```python
from build123d import *

# Parameters (mm, degrees)
SKETCH1_R           = 1
BOSS_EXTRUDE1_DEPTH = 3
SKETCH2_R           = 1.25
CUT_EXTRUDE1_DEPTH  = 4
SKETCH3_R           = 1.25
CUT_EXTRUDE2_DEPTH  = 4


with BuildPart() as part:
    # Sketch1 → Boss-Extrude1 (new body)
    with BuildSketch(Plane(origin=(0, 2.5, 0), x_dir=(1, 0, 0), z_dir=(0, 1, 0))):
        with BuildLine():
            Line((-2.5, -48.662329453), (-2.5, -18.662329453))
            ThreePointArc((-2.5, -18.662329453), (-5, -16.162329453), (-7.5, -18.662329453))
            Line((-7.5, -18.662329453), (-7.5, -48.662329453))
            ThreePointArc((-7.5, -48.662329453), (-5, -51.162329453), (-2.5, -48.662329453))
        make_face()
        with Locations((-5, -48.662329453)):
            Circle(SKETCH1_R, mode=Mode.SUBTRACT)
        with Locations((-5, -18.662329453)):
            Circle(SKETCH1_R, mode=Mode.SUBTRACT)
    extrude(amount=-BOSS_EXTRUDE1_DEPTH)

    # Sketch2 → Cut-Extrude1 (cut, through all)
    with BuildSketch(Plane.XZ.offset(0.5)):
        with Locations((-5, 18.662329453)):
            Circle(SKETCH2_R)
    extrude(amount=-CUT_EXTRUDE1_DEPTH, mode=Mode.SUBTRACT)

    # Sketch3 → Cut-Extrude2 (cut, through all)
    with BuildSketch(Plane.XZ.offset(0.5)):
        with Locations((-5, 48.662329453)):
            Circle(SKETCH3_R)
    extrude(amount=-CUT_EXTRUDE2_DEPTH, mode=Mode.SUBTRACT)


solid = part.part
```
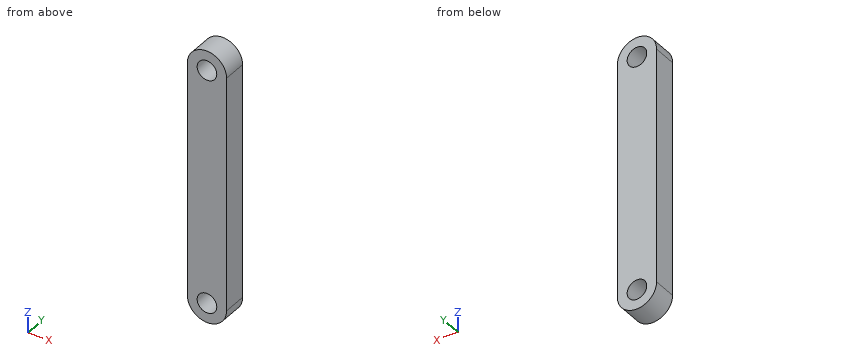
The model under review builds one solid part; all positions refer to its coordinate system, in mm. Round coordinates to 2 decimals unless told otherwise and drop trailing zeros. Loops run counter-clockwise (first coordinate to the right, second up) from the corner with the lowest first, then second, coordinate; pieces in that order, holes last. Notation, with made-up numbers: (39, -39) -> (71, -39) arc R18 ccw to (71, -15) -> close; hole circle Ø2 at (58.25, 9). An arc over 180 degrees is marked (long way). Answer in a Markdown table with one row per item.
1) Wall thickness on line 1 along Z through (x, y) = (-4.95, 0.05); line 2 along Z through (x, y) = (-4, 1.7); line 3 along X through (y, z) = (2.1, 48): over which ranges is each line inside the solid? List them lowest first.
Taken from the geometry:
| item | result |
|---|---|
| line 1 | z = 16.16 to 17.41, 19.91 to 47.41, 49.91 to 51.16 |
| line 2 | z = 16.37 to 17.91, 19.41 to 47.91, 49.41 to 50.95 |
| line 3 | x = -7.5 to -6.06, -3.94 to -2.5 |
2) Consider section C-C, the plane x = -3.1. Write out the cut boundary in (y, z).
Taken from the geometry:
| item | result |
|---|---|
| outline | (-0.5, 17.04) -> (2.5, 17.04) -> (2.5, 50.29) -> (-0.5, 50.29) -> close |
3) Consider section A-A, the plane x = -5. Write out the cut boundary in (y, z).
Taken from the geometry:
| item | result |
|---|---|
| outline | (-0.5, 16.16) -> (2.5, 16.16) -> (2.5, 17.41) -> (-0.5, 17.41) -> close; (-0.5, 19.91) -> (2.5, 19.91) -> (2.5, 47.41) -> (-0.5, 47.41) -> close; (-0.5, 49.91) -> (2.5, 49.91) -> (2.5, 51.16) -> (-0.5, 51.16) -> close |
4) Consider section B-B, the plane y = -0.2. Write out the cut boundary in (x, z).
Taken from the geometry:
| item | result |
|---|---|
| outline | (-7.5, 18.66) arc R2.5 ccw to (-2.5, 18.66) -> (-2.5, 48.66) arc R2.5 ccw to (-7.5, 48.66) -> close; hole circle Ø2.5 at (-5, 18.66); hole circle Ø2.5 at (-5, 48.66) |
